Here's how the part is built. I have some questions about the finished solid (model axes, mm). A direction names the side the tool comes from. Round coordinates to 2 decimals unless told otherwise and drop trailing zeros. Loops run counter-clockwise (first coordinate to the right, second up) from the corner with the lowest first, then second, coordinate; pieces in that order, holes last. Notation, with made-up numbers: M 24.5,11 L 33.5,11 A28 cw 33.5,32 Z; hole C 60.5,84 d2. An arc over 180 degrees is marked long. Answer as a JSON object with one key per item and string values.
from build123d import *

# Parameters (mm, degrees)
EXTRUDE_1_DEPTH        = 10
SKETCH_1_R             = 6
CUT_EXTRUDE_1_DEPTH    = 23
SKETCH_3_W             = 44
SKETCH_3_H             = 10
EXTRUDE_2_DEPTH        = 30
SKETCH_4_R             = 1.5
CUT_EXTRUDE_2_DEPTH    = 15
PATTERN_LINEAR_1_COUNT = 2
PATTERN_LINEAR_1_PITCH = 10
SKETCH_5_R             = 7.573705131
EXTRUDE_3_DEPTH        = 3
DRAFT_1_ANGLE          = 30


with BuildPart() as part:
    # 草图2 → 凸台-拉伸1 (new body)
    with BuildSketch(Plane.XY):
        with BuildLine():
            Line((-22, 75), (22, 75))
            Line((22, 75), (22, -21.471774194))
            add(Edge.make_bspline(
                [(-22, -21.471774194), (0, -49.899193548), (22, -21.471774194)],
                knots=[0, 0, 0, 1, 1, 1], degree=2))
            Line((-22, -21.471774194), (-22, 75))
        make_face()
    extrude(amount=EXTRUDE_1_DEPTH)

    # 草图1 → 切除-拉伸1 (cut)
    with BuildSketch(Plane.XY):
        Circle(SKETCH_1_R)
    extrude(amount=CUT_EXTRUDE_1_DEPTH, mode=Mode.SUBTRACT)

    # 草图3 → 凸台-拉伸2 (add)
    with BuildSketch(Plane.XY.offset(10)):
        with Locations((0, 70)):
            Rectangle(SKETCH_3_W, SKETCH_3_H)
    extrude(amount=EXTRUDE_2_DEPTH)

    # 草图4 → 切除-拉伸2 (cut)
    with BuildSketch(Plane(origin=(0, 75, 0), x_dir=(1, 0, 0), z_dir=(0, 1, 0))):
        with Locations((0, -32.875114596)):
            Circle(SKETCH_4_R)
    cut_extrude_2 = extrude(amount=-CUT_EXTRUDE_2_DEPTH, mode=Mode.SUBTRACT)

    # 阵列(线性)1: 切除-拉伸2 ×2
    with Locations(*[(-i * PATTERN_LINEAR_1_PITCH, 0, 0) for i in range(1, PATTERN_LINEAR_1_COUNT)]):
        add(cut_extrude_2, mode=Mode.SUBTRACT)

    # 草图5 → 凸台-拉伸3 (add)
    with BuildSketch(Plane.XY.offset(10)):
        Circle(SKETCH_5_R)
    extrude(amount=EXTRUDE_3_DEPTH)

    # 拔模1
    draft_1_faces = [part.faces().sort_by_distance(p)[0] for p in [
        (-7.573705131, 0, 11.5),
    ]]
    draft(draft_1_faces, Plane.XY.offset(13), DRAFT_1_ANGLE)


solid = part.part
Item 1: For P1, Ø13, axis at x = 0.5, y = -2, coming from the -Z side; P2, Ø5, axis at x = 0, z = 32.88, coming from the -Y side; P3, Ø16.5, axis at x = -0.5, y = -2.5, coming from the +Z side; P4, Ø8, axis at y = 60.5, z = 17, coming from the +X side, each with a flat end and sliding along its axis, tell me the tip position at first contact or that it passes through.
Solution:
{"P1": "stops at z = 0", "P2": "stops at y = 65", "P3": "stops at z = 13", "P4": "passes through"}
Item 2: I want a section at A-A on y = 0. List the corners of the cut face in (x, z) for me, plus the area to 3 significant figures.
Solution:
{"outline": "M -22,0 L -6,0 L -6,10 L 6,10 L 6,0 L 22,0 L 22,10 L 9.31,10 L 7.57,13 L -7.57,13 L -9.31,10 L -22,10 Z", "area": "371 mm2"}
Item 3: We'd pull the mould along Y, two halves only. Please class faces 3 (the face through (0, 75, 20)), 4 (the face through (-1.7, -7.5, 12.8)), 5 (the face through (0, 21, 10)), 6 (the face through (0, 0, 13)): +Y half, -Y half, draft (parallel to the pull), parting line (faces both ways), or undercut.
Solution:
{"face 3": "+Y half", "face 4": "undercut", "face 5": "undercut", "face 6": "draft"}
Item 4: I want a section at C-C on y = 60. List the corners of the cut face in (x, z) for me.
Solution:
{"outline": "M -22,0 L 22,0 L 22,10 L -22,10 Z"}
Item 5: I want a section at B-B on z = 16. List the corners of the cut face in (x, y) for me, plus the area to 3 significant figures.
Solution:
{"outline": "M -22,65 L 22,65 L 22,75 L -22,75 Z", "area": "440 mm2"}
Item 6: If I drill on L1, parallel to X at y = 0, z = 3.5; L2, parallel to Z at x = 12, y = -1.5; L3, parallel to Y at x = -7, z = 35.5, over which ranges is the centre line in solid material (lowest first)? Write a range as from..to.
Solution:
{"L1": "x = -22..-6, 6..22", "L2": "z = 0..10", "L3": "y = 65..75"}
Item 7: For faces 1 (the face through (0, 70, 40)), 2 (the face through (0, 0, 10)), which set-ups out of +Z, -Z, +X, -X, +Y, -Y let a thin tool reach every point of the face, with its end or its side?
Solution:
{"face 1": "+Z, +X, -X, +Y, -Y", "face 2": "-Z"}
